```python
from build123d import *


with BuildPart() as part:
    # 草图3 → 旋转1 (revolve)
    with BuildSketch(Plane(origin=(0, 0, 0), x_dir=(0, 0, -1), z_dir=(1, 0, 0))):
        Polygon((0, 0), (0, 175), (20, 175), (20, 67), (62.5, 67), (62.5, 6), (100, 6), (100, 0), align=None)
    revolve_1 = revolve(axis=Axis((0, 0, -100), (0, 0, 1)))

    # 镜向1: 旋转1 across plane
    add(revolve_1.mirror(Plane.XY))


solid = part.part
```
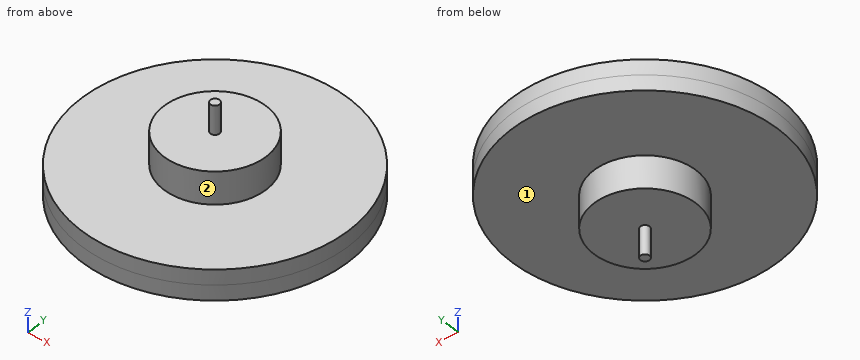
Can you work these out from the model? Positions are in its coordinate system, mm. Face numbers are marked on the shaded views. A direction names the side the tool comes from. Round coordinates to 2 decimals unless told otherwise and drop trailing zeros. Loops run counter-clockwise (first coordinate to the right, second up) from the corner with the lowest first, then second, coordinate; pieces in that order, holes last. Notation, with made-up numbers: M -0.5,-37 L 18.5,-37 A22 ccw 18.5,-3 Z; hole C 17,61 d4. An arc over 180 degrees is marked long. Answer in a Markdown table with one row per item.
1. On a 3-axis mill with a long thin cutter (end or side, diameter ignored), from which of +Z, -Z, +X, -X, +Y, -Y can I reach the whole of each face in a straight line? I mean the marked faces 1 and 2. Say none if no direction works.
Established:
| item | result |
|---|---|
| face 1 | -Z |
| face 2 | +Z |
2. If we section it at D-D, the plane z = -6: Please give me the cut outline in (x, y), plus the area to 3 significant figures.
Established:
| item | result |
|---|---|
| outline | C 0,0 d350 |
| area | 96,200 mm² |
3. If we section it at A-A, the plane y = 0: Please give me the cut outline in (x, z), plus the area to 3 significant figures.
Established:
| item | result |
|---|---|
| outline | M -175,-20 L -67,-20 L -67,-62.5 L -6,-62.5 L -6,-100 L 6,-100 L 6,-62.5 L 67,-62.5 L 67,-20 L 175,-20 L 175,20 L 67,20 L 67,62.5 L 6,62.5 L 6,100 L -6,100 L -6,62.5 L -67,62.5 L -67,20 L -175,20 Z |
| area | 26,300 mm² |
4. I'm going to push flat-ended pins straight in: pin 1 Ø5 at (y, z) = (-5, 44) entering from +X; pin 2 Ø1.5 at (y, z) = (37.5, 58) entering from -X; pin 3 Ø5 at (x, z) = (-42.5, 36.5) entering from -Y. Where does each tip first touch, or does it pass through?
Established:
| item | result |
|---|---|
| pin 1 | x = 66.95 |
| pin 2 | x = -56.02 |
| pin 3 | y = -53.75 |
5. Please list where these lines run through material, in increasing order: line 1 (Z direction, x = -42.5, y = 54); line 2 (Z direction, x = 54.5, y = -11); line 3 (Y direction, x = -110.5, z = 7). Write a range as from..to.
Established:
| item | result |
|---|---|
| line 1 | -20..20 |
| line 2 | -62.5..62.5 |
| line 3 | -135.7..135.7 |
6. If we section it at C-C, the plane z = -74.5: Please give me the cut outline in (x, y).
Established:
| item | result |
|---|---|
| outline | C 0,0 d12 |
